Geometry: final body of the model. Coordinates: model frame, mm. Face numbers are marked on the shaded views. A direction names the side the tool comes from. Give positions to 0.01 mm unless a question says otherwise; leave off trailing zeros. Order: outer loops, then holes, each group sorted by start corner. A loop starts at its lowest first (then second) coordinate and runs counter-clockwise, first axis right, second up. Notation, with made-up numbers: (16, -6) -> (41, -6) arc R3 ccw to (41, -2) -> close; hole circle Ø3 at (18, 62). An arc over 180 degrees is marked (long way). Answer in a Markdown table with one row per item. Add a question column.
Q1. Cut plane D-D on y = 14. Return the cut outline in (x, z).
Q2. Set-up query: the marked faces 1, 2 and 3. Return all of +Z, -Z, +X, -X, +Y, -Y with unobstructed straight access to the full face (end or side cutting, diameter ignored); none if empty.
Q3. Pull-direction query (X, two-part tool) for the marked faces 4, 5, 6 and 7; classes: +X half, -X half, draft (parallel to the pull), parting line (faces both ways), or undercut.
Q4. Cut plane B-B on x = -34. Return the cut outline in (y, z), and give its area (3 significant figures).
Q5. Line query: line 1 along Z through (x, y) = (-34, 3); line 2 along X through (y, z) = (3, 10.5); line 3 along X through (y, z) = (44, 14.5). Output: solid intervals per line, ascending. Write a range as from..to.
Q6. Contact query for flat-ended pins moving along their axis: P1, Ø1, axis at y = 12, z = 12.5, coming from the -X side; P2, Ø1, axis at y = 21, z = 6.5, coming from the +X side; P3, Ø1, axis at y = 36.5, z = 2.5, coming from the -X side; P4, Ø6, axis at x = -9, z = 11, coming from the +Y side. Output: stop coordinate, or through.
from build123d import *

# Parameters (mm, degrees)
F1_DEPTH  = 20
F2_W      = 9
F2_H      = 20
F2_W_2    = 20
F2_H_2    = 9
F3_DEPTH  = 1.5
F4_W      = 40
F4_H      = 9
F4_W_2    = 9
F4_H_2    = 20
F5_DEPTH  = 1.5
F6_SIZE   = 1.49999
F7_R      = 2.65
F8_DEPTH  = 5.5
F9_R      = 2.65
F10_DEPTH = 5.5


# Not quite as in the source:
# - a fillet or chamfer is up to 0.001 mm smaller than in the source, because OpenCascade refuses the exact size


with BuildPart() as f1:
    # F0 (on Top) → F1 (new body)
    with BuildSketch(Plane.XY):
        Polygon((-64, 0), (0, 0), (0, 64), (-4, 64), (-4, 4), (-64, 4), align=None)
    extrude(amount=F1_DEPTH)

    # F2 (on face) → F3 (join)
    with BuildSketch(Plane(origin=(0, 4, 0), x_dir=(-1, 0, 0), z_dir=(0, 1, 0))):
        with Locations((14, 10)):
            Rectangle(F2_W, F2_H)
        with Locations((34, 10)):
            Rectangle(F2_W, F2_H)
        with Locations((54, 10)):
            Rectangle(F2_W_2, F2_H_2)
    extrude(amount=F3_DEPTH)

    # F4 (on face) → F5 (join)
    with BuildSketch(Plane(origin=(-4, 0, 0), x_dir=(0, -1, 0), z_dir=(-1, 0, 0))):
        with Locations((-44, 10)):
            Rectangle(F4_W, F4_H)
        with Locations((-14, 10)):
            Rectangle(F4_W_2, F4_H_2)
    extrude(amount=F5_DEPTH)

    # F6 (size 1.5 in the source; OpenCascade refuses exactly that, so slightly less here)
    f6_edges = [f1.edges().sort_by_distance(p)[0] for p in [
        (-5.5, 64, 10),
        (-5.5, 44, 14.5),
        (-5.5, 44, 5.5),
        (-5.5, 24, 10),
        (-54, 5.5, 14.5),
        (-54, 5.5, 5.5),
        (-44, 5.5, 10),
        (-64, 5.5, 10),
        (-34, 5.5, 20),
        (-29.5, 5.5, 10),
        (-34, 5.5, 0),
        (-38.5, 5.5, 10),
        (-14, 5.5, 20),
        (-9.5, 5.5, 10),
        (-14, 5.5, 0),
        (-18.5, 5.5, 10),
        (-5.5, 9.5, 10),
        (-5.5, 14, 20),
        (-5.5, 18.5, 10),
        (-5.5, 14, 0),
    ]]
    chamfer(f6_edges, length=F6_SIZE)

    # F7 (on face) → F8 (cut, through all)
    with BuildSketch(Plane(origin=(0, 5.5, 0), x_dir=(-1, 0, 0), z_dir=(0, 1, 0))):
        with Locations((14, 10)):
            Circle(F7_R)
        with Locations((34, 10)):
            Circle(F7_R)
        with Locations((54, 10)):
            Circle(F7_R)
    extrude(amount=-F8_DEPTH, mode=Mode.SUBTRACT)

    # F9 (on face) → F10 (cut, through all)
    with BuildSketch(Plane(origin=(-5.5, 0, 0), x_dir=(0, -1, 0), z_dir=(-1, 0, 0))):
        with Locations((-54, 10)):
            Circle(F9_R)
        with Locations((-34, 10)):
            Circle(F9_R)
        with Locations((-14, 10)):
            Circle(F9_R)
    extrude(amount=-F10_DEPTH, mode=Mode.SUBTRACT)


solid = f1.part
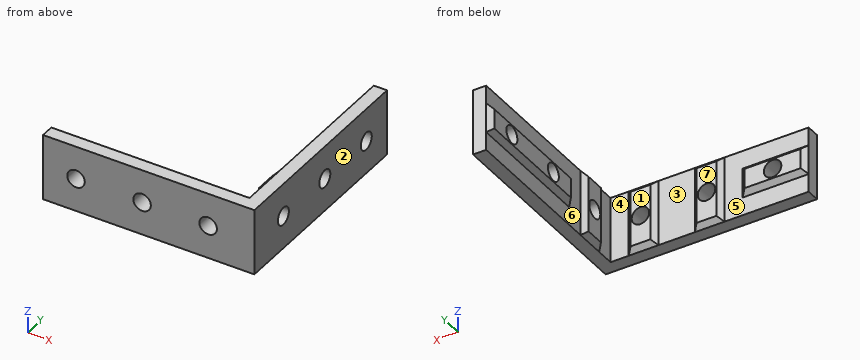
Completed:
| question | item | result |
|---|---|---|
| 1 | outline | (-5.5, 1.5) -> (-4, 0) -> (0, 0) -> (0, 7.35) -> (-5.5, 7.35) -> close; (-5.5, 12.65) -> (0, 12.65) -> (0, 20) -> (-4, 20) -> (-5.5, 18.5) -> close |
| 2 | face 1 | +Z, -Z, -X, +Y |
| 2 | face 2 | +Z, -Z, +X, +Y, -Y |
| 2 | face 3 | +Z, -Z, +Y |
| 3 | face 4 | undercut |
| 3 | face 5 | undercut |
| 3 | face 6 | -X half |
| 3 | face 7 | draft |
| 4 | outline | (0, 0) -> (4, 0) -> (5.5, 1.5) -> (5.5, 7.35) -> (0, 7.35) -> close; (0, 12.65) -> (5.5, 12.65) -> (5.5, 18.5) -> (4, 20) -> (0, 20) -> close |
| 4 | area | 78.6 mm² |
| 5 | line 1 | z = 0..7.35, 12.65..20 |
| 5 | line 2 | x = -64..-56.6, -51.4..-36.6, -31.4..-16.6, -11.4..0 |
| 5 | line 3 | x = -4..0 |
| 6 | P1 | stops at x = -5.5 |
| 6 | P2 | stops at x = 0 |
| 6 | P3 | stops at x = -4 |
| 6 | P4 | stops at y = 5.5 |
